Autodesk Inventor part; units mm, degrees
ref_plane "YZ Plane" through (0, 0, 0) normal (1, 0, 0) x (0, 1, 0)
ref_plane "XZ Plane" through (0, 0, 0) normal (0, 1, 0) x (-1, 0, 0)
ref_plane "XY Plane" through (0, 0, 0) normal (0, 0, 1) x (1, 0, 0)
sketch "Sketch1" plane through (0, 0, 0) normal (0, 1, 0) x (-1, 0, 0)
  circle A0 centre (0, 0) radius 300
  dimension "d0" = 600
extrude "Extrusion1" add sketch "Sketch1" along normal blind 75
sketch "Sketch2" plane through (0, 75, 0) normal (0, 1, 0) x (1, 0, 0)
  circle A0 centre (0, 0) radius 250
  dimension "d3" = 500
extrude "Extrusion2" add sketch "Sketch2" along normal blind 75
loft "Loft1" add section 1 edges at (-250, 150, 0) section 2 edges at (300, 75, 0)
fillet "Fillet1" radius 4 1 edges at (-250, 150, 0)
fillet "Fillet2" radius 4 2 edges at (0, 75, -300) (0, 75, 300)
properties part number "Base"
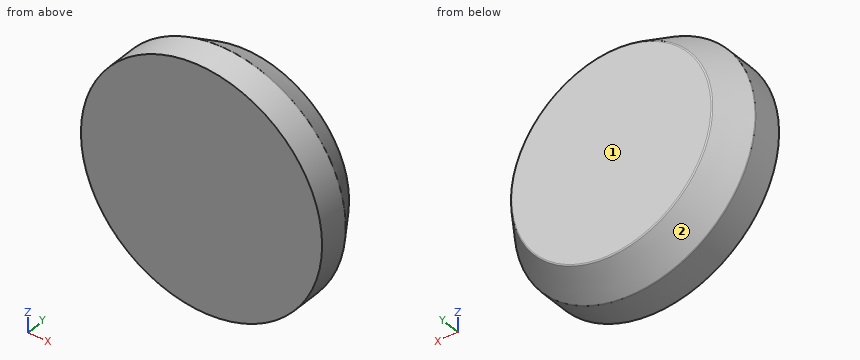
The model under review builds one solid part; all positions refer to its coordinate system, in mm. Face numbers are marked on the shaded views. Round coordinates to 2 decimals unless told otherwise and drop trailing zeros. Write each loop counter-clockwise with the first axis right and the second up, starting at its lowest first coordinate (ties: lowest second). Pieces come first, ordered by that corner, then holes.
(1) Mouldability with a two-part tool opening along Z and no side actions: class the marked faces 1 and 2 as +Z half, -Z half, draft (parallel to the pull), parting line (faces both ways), or undercut.
(2) We need section A-A on y = 115. Give the boundary of the cut face in (x, z).
(3) Insertion check: pin 1 (12 mm diameter, centred on y = 126.5, z = 98.5, fed in from +X); pin 2 (2 mm diameter, centred on x = 104, y = 114, fed in from +Z); pin 3 (6 mm diameter, centred on y = 88.5, z = -210.5, fed in from -X). Each pin has a flat end and moves straight along its axis. Give the tip position at first contact, or say it passes through.
(4) Wall thickness on L1, parallel to X at y = 9.5, z = 133.5; L2, parallel to Z at x = -203, y = 109; L3, parallel to Z at x = 29, y = 52.5: over which ranges is each line inside the solid? List them lowest first.
Findings below:
1. face 1: draft
1. face 2: parting line
2. outline: circle Ø546.67 at (0, 0)
3. pin 1: stops at x = 251.62
3. pin 2: stops at z = 254.32
3. pin 3: stops at x = -205.15
4. L1: x = -268.66 to 268.66
4. L2: z = -188.96 to 188.96
4. L3: z = -298.6 to 298.6
